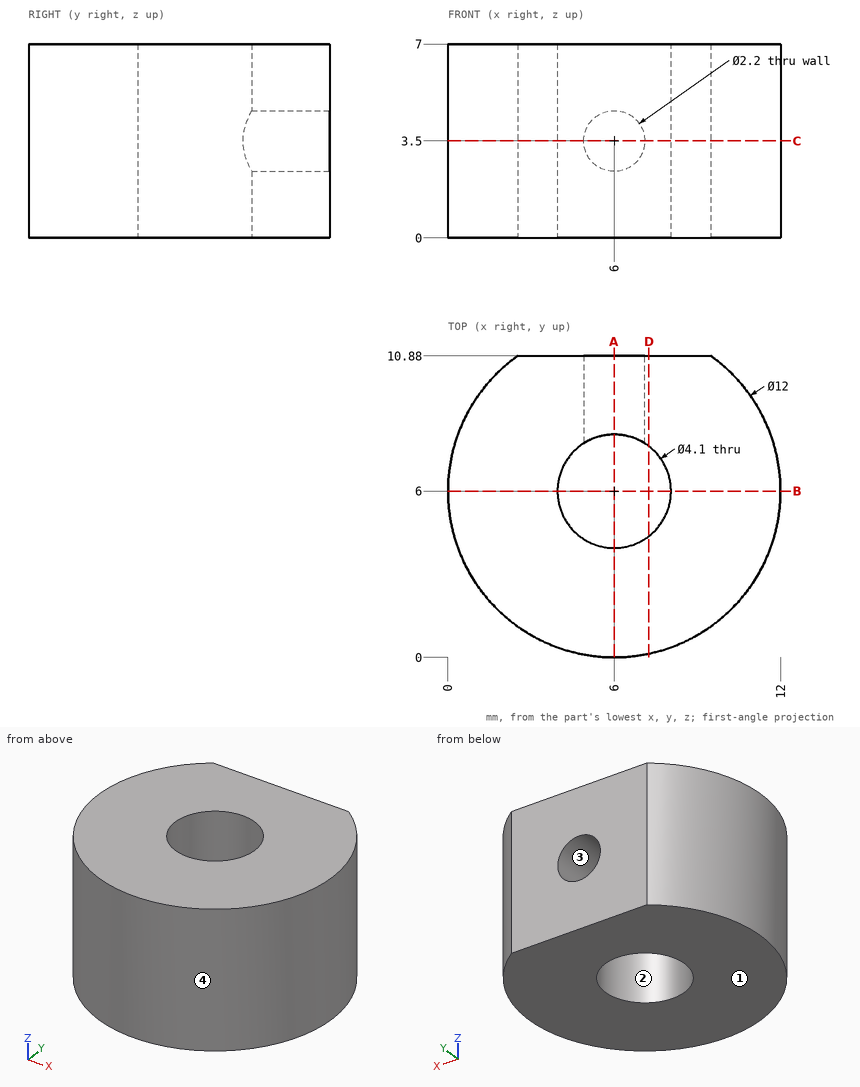
Design review of the part shown in the three views and the two pictorial views. Dimensions are in mm from the part's minimum x, y and z. Round coordinates to 2 decimals unless told otherwise and drop trailing zeros. Write each loop counter-clockwise with the first axis right and the second up, starting at its lowest first coordinate (ties: lowest second). Pieces come first, ordered by that corner, then holes.
1) For line 1 along Y through (x, z) = (6, 2.25); line 2 along Z through (x, y) = (6, 9.6); line 3 along Y through (x, z) = (6, 3.75), list the stretches that pass through material, from the lowest coordinate up.
Answer below:
line 1: y = 0 to 3.95, 8.05 to 10.88
line 2: z = 0 to 2.4, 4.6 to 7
line 3: y = 0 to 3.95
2) Take a section at B-B on y = 6. Give the boundary of the cut face in (x, z), then the cut area to 3 significant figures.
Answer below:
outline: (0, 0) - (3.95, 0) - (3.95, 7) - (0, 7) - close; (8.05, 0) - (12, 0) - (12, 7) - (8.05, 7) - close
area: 55.3 mm2
3) Insertion check: pin 1 Ø1 at (y, z) = (8, 6) entering from -X; pin 2 Ø4.5 at (x, y) = (6, 6) entering from +Z; pin 3 Ø3 at (y, z) = (9.5, 2) entering from -X; pin 4 Ø3 at (y, z) = (8.5, 3) entering from +X. Each pin has a flat end and moves straight along its axis. Give the tip position at first contact, or say it passes through.
Answer below:
pin 1: stops at x = 0.19
pin 2: stops at z = 7
pin 3: stops at x = 0.34
pin 4: stops at x = 11.92
4) Take a section at D-D on x = 7.25. Give the boundary of the cut face in (y, z) (1 decimal), then the cut area to 3 significant figures.
Answer below:
outline: (0.1, 0) - (4.4, 0) - (4.4, 7) - (0.1, 7) - close; (7.6, 0) - (10.9, 0) - (10.9, 7) - (7.6, 7) - close
area: 52.5 mm2
5) Take a section at A-A on x = 6. Give the boundary of the cut face in (y, z).
Answer below:
outline: (0, 0) - (3.95, 0) - (3.95, 7) - (0, 7) - close; (8.05, 0) - (10.88, 0) - (10.88, 2.4) - (8.05, 2.4) - close; (8.05, 4.6) - (10.88, 4.6) - (10.88, 7) - (8.05, 7) - close
6) Take a section at C-C on z = 3.5. Give the boundary of the cut face in (x, y).
Answer below:
outline: (2.51, 10.88) arc R6 ccw (long way) to (9.49, 10.88) - (7.1, 10.88) - (7.1, 7.73) arc R2.05 cw (long way) to (4.9, 7.73) - (4.9, 10.88) - close
7) Mouldability with a two-part tool opening along X and no side actions: class the marked faces 1, 2, 3 and 4 as +X half, -X half, draft (parallel to the pull), parting line (faces both ways), or undercut.
Answer below:
face 1: draft
face 2: undercut
face 3: undercut
face 4: parting line
